```python
from build123d import *

# Parameters (mm, degrees)
SKETCH2_R                                     = 1
BOSS_EXTRUDE3_DEPTH                           = 1.5875
DB15_PLUG_CUTAWAY_DEPTH                       = 55.106562968
CSK_FOR_4_FLAT_HEAD_MACHINE_SCREW1_AT_2_COUNT = 2
CSK_FOR_4_FLAT_HEAD_MACHINE_SCREW1_AT_2_PITCH = 51.65
CSK_FOR_4_FLAT_HEAD_MACHINE_SCREW1_AT_3_COUNT = 2
CSK_FOR_4_FLAT_HEAD_MACHINE_SCREW1_AT_3_PITCH = 81.65
CSK_FOR_4_FLAT_HEAD_MACHINE_SCREW1_AT_4_COUNT = 2
CSK_FOR_4_FLAT_HEAD_MACHINE_SCREW1_AT_4_PITCH = 96.614931558
SKETCH11_R                                    = 1.7399
CUT_EXTRUDE1_DEPTH                            = 55.106562968


with BuildPart() as part:
    # Sketch2 → Boss-Extrude3 (new body)
    with BuildSketch(Plane(origin=(0, 0, 0), x_dir=(1, 0, 0), z_dir=(0, 1, 0))):
        with BuildLine():
            Line((-45, 25.825), (-45, -25.825))
            ThreePointArc((-45, -25.825), (-43.777170811, -28.777170811), (-40.825, -30))
            Line((-40.825, -30), (40.825, -30))
            ThreePointArc((40.825, -30), (43.777170811, -28.777170811), (45, -25.825))
            Line((45, -25.825), (45, 25.825))
            ThreePointArc((45, 25.825), (43.777170811, 28.777170811), (40.825, 30))
            Line((40.825, 30), (-40.825, 30))
            ThreePointArc((-40.825, 30), (-43.777170811, 28.777170811), (-45, 25.825))
        make_face()
        with Locations(Location((40.825, 25.825, 0), (0, 0, 270))):
            Circle(SKETCH2_R, mode=Mode.SUBTRACT)
        with Locations(Location((-40.825, 25.825, 0), (0, 0, 270))):
            Circle(SKETCH2_R, mode=Mode.SUBTRACT)
        with Locations(Location((-40.825, -25.825, 0), (0, 0, 270))):
            Circle(SKETCH2_R, mode=Mode.SUBTRACT)
        with Locations(Location((40.825, -25.825, 0), (0, 0, 270))):
            Circle(SKETCH2_R, mode=Mode.SUBTRACT)
    extrude(amount=BOSS_EXTRUDE3_DEPTH)

    # Sketch4 → DB15 Plug Cutaway (cut, through all)
    with BuildSketch(Plane.XZ):
        with BuildLine():
            Line((-13.835, 6.924614493), (-13.835, 11.090214492))
            ThreePointArc((-13.835, 11.090214492), (-12.684222543, 13.868437036), (-9.905999998, 15.019214492))
            Line((-9.905999998, 15.019214492), (9.905999999, 15.019214492))
            ThreePointArc((9.905999999, 15.019214492), (12.684222543, 13.868437035), (13.835, 11.090214492))
            Line((13.835, 11.090214492), (13.835, 6.924614492))
            ThreePointArc((13.835, 6.924614492), (12.684222543, 4.146391949), (9.906, 2.995614492))
            Line((9.906, 2.995614492), (-9.905999998, 2.995614492))
            ThreePointArc((-9.905999998, 2.995614492), (-12.684222543, 4.146391948), (-13.835, 6.924614493))
        make_face()
    extrude(amount=-DB15_PLUG_CUTAWAY_DEPTH, mode=Mode.SUBTRACT)

    # Sketch9 → CSK for #4 Flat Head Machine Screw1 (revolve, cut)
    with BuildSketch(Plane(origin=(-40.825, 0, 25.825), x_dir=(0, 0, -1), z_dir=(1, 0, 0))):
        Polygon((0, 0), (0, 1.5875), (1.63195, 1.5875), (1.63195, 1.409834001), (2.8575, 0), align=None)
    csk_for_4_flat_head_machine_screw1 = revolve(axis=Axis((-40.825, -6.35, 25.825), (0, 1, 0)), mode=Mode.SUBTRACT)

    # CSK for #4 Flat Head Machine Screw1 at 2: CSK for #4 Flat Head Machine Screw1 ×2
    with Locations(*[(0, 0, -i * CSK_FOR_4_FLAT_HEAD_MACHINE_SCREW1_AT_2_PITCH) for i in range(1, CSK_FOR_4_FLAT_HEAD_MACHINE_SCREW1_AT_2_COUNT)]):
        add(csk_for_4_flat_head_machine_screw1, mode=Mode.SUBTRACT)

    # CSK for #4 Flat Head Machine Screw1 at 3: CSK for #4 Flat Head Machine Screw1 ×2
    with Locations(*[(i * CSK_FOR_4_FLAT_HEAD_MACHINE_SCREW1_AT_3_PITCH, 0, 0) for i in range(1, CSK_FOR_4_FLAT_HEAD_MACHINE_SCREW1_AT_3_COUNT)]):
        add(csk_for_4_flat_head_machine_screw1, mode=Mode.SUBTRACT)

    # CSK for #4 Flat Head Machine Screw1 at 4: CSK for #4 Flat Head Machine Screw1 ×2
    with Locations(*[Vector(0.8451074661352507, 0, -0.5345964559202167) * (i * CSK_FOR_4_FLAT_HEAD_MACHINE_SCREW1_AT_4_PITCH) for i in range(1, CSK_FOR_4_FLAT_HEAD_MACHINE_SCREW1_AT_4_COUNT)]):
        add(csk_for_4_flat_head_machine_screw1, mode=Mode.SUBTRACT)

    # Sketch11 → Cut-Extrude1 (cut, through all)
    with BuildSketch(Plane.XZ):
        with Locations(Location((-30.382, -0.009017528, 0), (0, 0, 270))):
            Circle(SKETCH11_R)
        with Locations(Location((30.382, -0.061487226, 0), (0, 0, 270))):
            Circle(SKETCH11_R)
    extrude(amount=-CUT_EXTRUDE1_DEPTH, mode=Mode.SUBTRACT)


solid = part.part
```
Geometry check sheet. Reference: the model listing, model coordinates, mm. A direction names the side the tool comes from. Round coordinates to 2 decimals unless told otherwise and drop trailing zeros. Order: outer loops, then holes, each group sorted by start corner. A loop starts at its lowest first (then second) coordinate and runs counter-clockwise, first axis right, second up. Notation, with made-up numbers: (71.25, -11) - (110.25, -11) arc R21 cw to (110.25, 20) - close; hole circle Ø11 at (-26, 85). An arc over 180 degrees is marked (long way). Use a Markdown table: item, result. Add a question column.
1) Section check A-A (z = 10). Record the cut outline in (x, y) (1 decimal).
2) Gauge pin test, flat ends, axial feed: P1, Ø3, axis at x = 40.825, z = -25.825, coming from the +Y side; P2, Ø8, axis at x = -32, z = -19.5, coming from the -Y side. Record the tip position at first contact, or that the pin passes through.
3) Thickness scan on line 1 along Z through (x, y) = (0, 0.7); line 2 along X through (y, z) = (1.1, 8.5) (3 decimals); line 3 along X through (y, z) = (1, 4.5). Record the ranges inside material, lowest first.
4) Mould release check, pull along X, two halves, no side actions. Record for faces 3 (the cylindrical face through (-31.926, 0.783, -0.812)), 4 (the flat face through (-1, 1.588, 0)), 5 (the cylindrical face through (-43.809, 0.783, 28.745)): released by +X, released by -X, zero draft, split by the parting line, or undercut.
5) Section check B-B (x = -7.5). Record the cut outline in (y, z), then the cut area to 3 significant figures.
6) Section check C-C (y = 0.85). Record the cut outline in (x, z) (3 decimals), then the cut area to 3 significant figures.
7) Set-up check for faces 1 (the cylindrical face through (43.809, 0.783, -28.745)), 2 (the cylindrical face through (-12.654, 0.783, 4.116)): record each of +Z, -Z, +X, -X, +Y, -Y from which the full face is reachable in a straight line by a thin tool's end or side.
Established:
| question | item | result |
|---|---|---|
| 1 | outline | (-45, 0) - (-13.8, 0) - (-13.8, 1.6) - (-45, 1.6) - close; (13.8, 0) - (45, 0) - (45, 1.6) - (13.8, 1.6) - close |
| 2 | P1 | through |
| 2 | P2 | y = 0 |
| 3 | line 1 | -30 to 3, 15.02 to 30 |
| 3 | line 2 | -45 to -13.835, 13.835 to 45 |
| 3 | line 3 | -45 to -13, 13 to 45 |
| 4 | face 3 | undercut |
| 4 | face 4 | zero draft |
| 4 | face 5 | released by -X |
| 5 | outline | (0, -30) - (1.59, -30) - (1.59, 3) - (0, 3) - close; (0, 15.02) - (1.59, 15.02) - (1.59, 30) - (0, 30) - close |
| 5 | area | 76.2 mm2 |
| 6 | outline | (-45, -25.825) arc R4.175 ccw to (-40.825, -30) - (40.825, -30) arc R4.175 ccw to (45, -25.825) - (45, 25.825) arc R4.175 ccw to (40.825, 30) - (-40.825, 30) arc R4.175 ccw to (-45, 25.825) - close; hole circle Ø4.237 at (-40.825, -25.825); hole circle Ø4.237 at (-40.825, 25.825); hole circle Ø3.48 at (-30.382, -0.009); hole (-13.835, 6.925) arc R3.929 ccw to (-9.906, 2.996) - (9.906, 2.996) arc R3.929 ccw to (13.835, 6.925) - (13.835, 11.09) arc R3.929 ccw to (9.906, 15.019) - (-9.906, 15.019) arc R3.929 ccw to (-13.835, 11.09) - close; hole circle Ø3.48 at (30.382, -0.061); hole circle Ø4.237 at (40.825, -25.825); hole circle Ø4.237 at (40.825, 25.825) |
| 6 | area | 4,990 mm2 |
| 7 | face 1 | -Z, +X, +Y, -Y |
| 7 | face 2 | +Y, -Y |
